Print and shaded views of the part. All mm, measured from the part's lowest x, y and z. Give positions to 0.01 mm unless a question says otherwise; leave off trailing zeros. Write each loop counter-clockwise with the first axis right and the second up, starting at its lowest first coordinate (ties: lowest second). Pieces come first, ordered by that corner, then holes. Notation, with made-up numbers: (39.25, 64) -> (51.25, 64) arc R14 ccw to (51.25, 87) -> close; hole circle Ø7 at (88, -16.5). An arc over 180 degrees is marked (long way). Put each result on its own line as item: value.
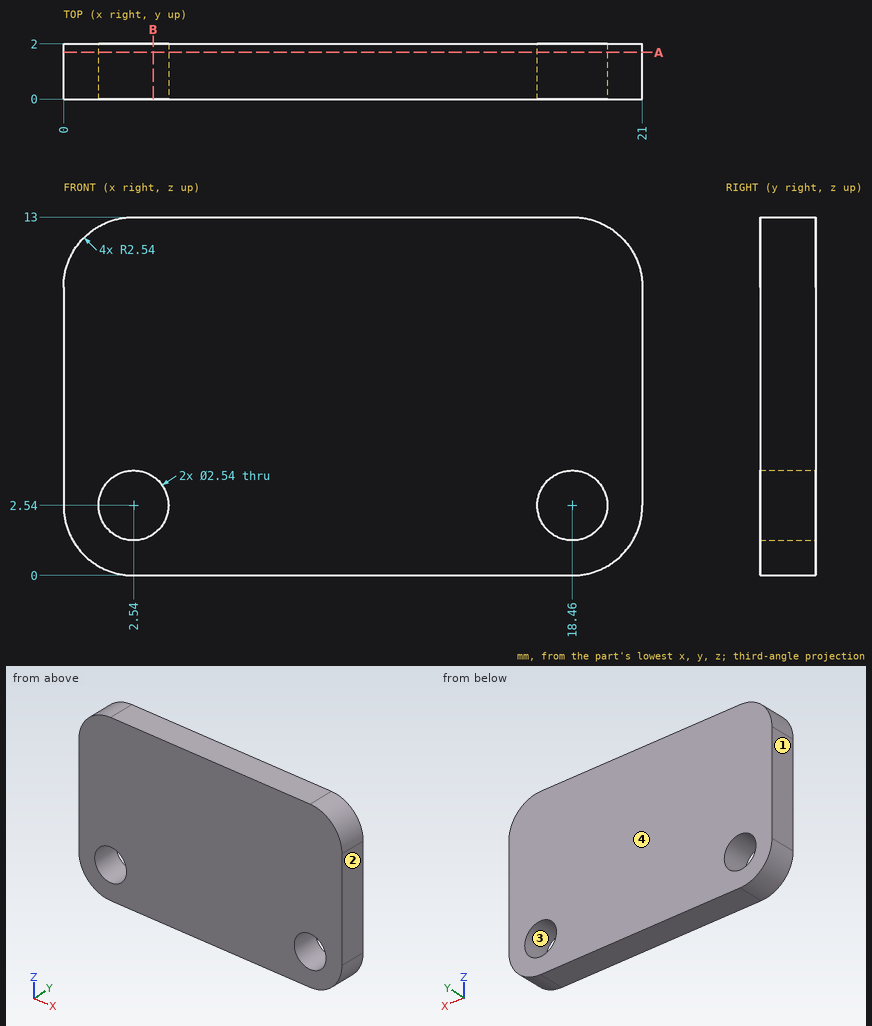
1) Wall check: L1, parallel to X at y = 1.45, z = 2.54; L2, parallel to Z at x = 2.54, y = 0.85; L3, parallel to Z at x = 3, y = 0.15. Give the ranges that are in metal, low to high.
Filled sheet:
L1: 0 to 1.27, 3.81 to 17.19, 19.73 to 21
L2: 0 to 1.27, 3.81 to 13
L3: 0 to 1.36, 3.72 to 13
2) Slice it at A-A (y = 1.7). Write the cut outline in (x, z), plus the area to 3 significant figures.
Filled sheet:
outline: (0, 2.54) arc R2.54 ccw to (2.54, 0) -> (18.46, 0) arc R2.54 ccw to (21, 2.54) -> (21, 10.46) arc R2.54 ccw to (18.46, 13) -> (2.54, 13) arc R2.54 ccw to (0, 10.46) -> close; hole circle Ø2.54 at (2.54, 2.54); hole circle Ø2.54 at (18.46, 2.54)
area: 257 mm2
3) Slice it at B-B (x = 3.25). Write the cut outline in (y, z).
Filled sheet:
outline: (0, 0) -> (2, 0) -> (2, 1.49) -> (0, 1.49) -> close; (0, 3.59) -> (2, 3.59) -> (2, 13) -> (0, 13) -> close
4) Pull direction X, two halves, no side cores. Call the marked faces 1, 2, 3 and 4: released by +X, released by -X, zero draft, split by the parting line, or undercut.
Filled sheet:
face 1: released by -X
face 2: released by +X
face 3: undercut
face 4: zero draft
